Can you work these out from the model? Positions are in its coordinate system, mm. A direction names the side the tool comes from. Coordinates: 2 decimals unless noted, no trailing zeros. Order: outer loops, then holes, each group sorted by start corner. A loop starts at its lowest first (then second) coordinate and runs counter-clockwise, first axis right, second up.
```python
from build123d import *

# Parameters (mm, degrees)
F0_W     = 12.7
F0_H     = 76.2
F1_DEPTH = 114.3
F3_DEPTH = 12.7
F4_W     = 228.6
F4_H     = 6.35
F5_DEPTH = 4.7625


with BuildPart() as f1:
    # F0 (on Front) → F1 (new body, symmetric)
    with BuildSketch(Plane.XZ):
        Rectangle(F0_W, F0_H)
    extrude(amount=F1_DEPTH, both=True)

    # F2 (on face) → F3 (cut, through all)
    with BuildSketch(Plane.YZ.offset(6.35)):
        Polygon((-101.6, 25.4), (-114.3, 25.4), (-114.3, 15.875), (-101.6, 13.33729), align=None)
        Polygon((-114.3, -28.575), (-114.3, -38.1), (-101.6, -38.1), (-101.6, -26.03729), align=None)
        Polygon((114.3, 28.575), (114.3, 38.1), (101.6, 38.1), (101.6, 26.03729), align=None)
        Polygon((101.6, -38.1), (114.3, -38.1), (114.3, -28.575), (101.6, -26.03729), align=None)
    extrude(amount=-F3_DEPTH, mode=Mode.SUBTRACT)

    # F4 (on face) → F5 (cut)
    with BuildSketch(Plane.YZ.offset(6.35)):
        with Locations((0, 28.575)):
            Rectangle(F4_W, F4_H)
    extrude(amount=-F5_DEPTH, mode=Mode.SUBTRACT)


solid = f1.part
```
1. I'm going to push flat-ended pins straight in: pin 1 (1.9 mm diameter, centred on y = -47.5, z = 28, fed in from +X); pin 2 (6 mm diameter, centred on x = 2, z = 19.5, fed in from -Y); pin 3 (3.5 mm diameter, centred on x = -2.5, z = 32, fed in from +Y). Where does each tip first touch, or does it pass through?
Completed:
pin 1: stops at x = 1.59
pin 2: stops at y = -101.6
pin 3: stops at y = 101.6
2. Thinking about a two-plate mould opening in Z: for faces 1 (the flat face through (-2.33, 107.86, 27.29)), 2 (the flat face through (-2, -108, 25.4)), 3 (the flat face through (6.35, -2, -7)), which applies, pulls with the +Z half, pulls with the -Z half, needs draft (parallel to the pull), parting line crosses it, or undercut?
Completed:
face 1: pulls with the +Z half
face 2: undercut
face 3: needs draft
3. Imagine slicing it at B-B on y = 22.5. Please give me the cut outline in (x, z), then the cut area to 4 significant figures.
Completed:
outline: (-6.35, -38.1) - (6.35, -38.1) - (6.35, 25.4) - (1.59, 25.4) - (1.59, 31.75) - (6.35, 31.75) - (6.35, 38.1) - (-6.35, 38.1) - close
area: 937.5 mm2
4. Imagine slicing it at A-A on x = -3. Please give me the cut outline in (y, z) (3 decimals).
Completed:
outline: (-114.3, -28.575) - (-101.6, -26.037) - (-101.6, -38.1) - (101.6, -38.1) - (101.6, -26.037) - (114.3, -28.575) - (114.3, 28.575) - (101.6, 26.037) - (101.6, 38.1) - (-114.3, 38.1) - (-114.3, 25.4) - (-101.6, 25.4) - (-101.6, 13.337) - (-114.3, 15.875) - close
5. On a 3-axis mill with a long thin cutter (end or side, diameter ignored), from which of +Z, -Z, +X, -X, +Y, -Y can I reach the whole of each face in a straight line? I mean faces 4 (the flat face through (0.089, -108.039, 14.624)), 5 (the flat face through (4, 5, 25.4)), 6 (the flat face through (0.089, 108.039, -27.324)), 7 (the flat face through (0, -8, 38.1)), 8 (the flat face through (-1, 101.6, 32)). Say none if no direction works.
Completed:
face 4: +X, -X
face 5: +X, +Y, -Y
face 6: -Z, +X, -X
face 7: +Z, +X, -X, +Y, -Y
face 8: +Z, +X, -X
6. Please list where these lines run through material, in increasing order: probe 1 along Z at (x, y) = (4.75, -41.5); probe 2 along Y at (x, z) = (-2.25, 31.5); probe 3 along Y at (x, z) = (3.25, 21.5).
Completed:
probe 1: z = -38.1 to 25.4, 31.75 to 38.1
probe 2: y = -114.3 to 101.6
probe 3: y = -101.6 to 114.3
